Geometry: final body of the model. Coordinates: model frame, mm. A direction names the side the tool comes from. Coordinates: 2 decimals unless noted, no trailing zeros. Order: outer loops, then holes, each group sorted by start corner. A loop starts at its lowest first (then second) coordinate and runs counter-clockwise, first axis right, second up. Notation, with made-up numbers: (-21.5, 59.5) -> (-5.5, 59.5) arc R26 ccw to (-5.5, 87.5) -> close; hole circle Ø9 at (73, 20.25). An arc over 180 degrees is marked (long way). Answer in a Markdown table with one row per item. Add a question column.
1) Ray query, line 1 (X direction, y = 1.8, z = -44); line 2 (Z direction, x = -37, y = 0.65). Return the intervals inside material, ascending. Write a range as from..to.
2) Section query A-A on y = 1.45. Return the cut outline in (x, z) (3 decimals), then the cut area to 3 significant figures.
3) Section query B-B on x = -50.5. Return the cut outline in (y, z) (3 decimals), then the cut area to 3 significant figures.
4) Section query C-C on z = -39.5. Return the cut outline in (x, y) (3 decimals).
5) Contact query for flat-ended pins moving along their axis: P1, Ø1, axis at y = 2, z = -95, coming from the +X side; P2, Ø1, axis at y = 2, z = -81, coming from the -X side; P3, Ø12, axis at x = 17.5, z = -91.5, coming from the -Y side. Output: stop coordinate, or through.
6) Set-up query: faces 1 (the face through (32, 2, 0)), 2 (the face through (59.31, 1.57, 3.24)), 3 (the face through (-6.35, 2, -77)). Return all of +Z, -Z, +X, -X, +Y, -Y with unobstructed straight access to the full face (end or side cutting, diameter ignored); none if empty.
```python
from build123d import *

# Parameters (mm, degrees)
BOSS_EXTRUDE1_DEPTH = 3.175


with BuildPart() as part:
    # Sketch1 → Boss-Extrude1 (new body)
    with BuildSketch(Plane(origin=(0, 0, 0), x_dir=(1, 0, 0), z_dir=(0, 1, 0))):
        with BuildLine():
            Line((-6.35, 0), (-56.134, 0))
            ThreePointArc((-56.134, 0), (-59.309, -3.175), (-56.134, -6.35))
            Line((-56.134, -6.35), (56.134, -6.35))
            ThreePointArc((56.134, -6.35), (59.309, -3.175), (56.134, 0))
            Line((56.134, 0), (6.35, 0))
            Line((6.35, 0), (6.35, 152.4))
            Line((6.35, 152.4), (-6.35, 152.4))
            Line((-6.35, 152.4), (-6.35, 0))
        make_face()
    extrude(amount=BOSS_EXTRUDE1_DEPTH)


solid = part.part
```
Result:
| question | item | result |
|---|---|---|
| 1 | line 1 | -6.35..6.35 |
| 1 | line 2 | 0..6.35 |
| 2 | outline | (-56.134, 0) -> (-6.35, 0) -> (-6.35, -152.4) -> (6.35, -152.4) -> (6.35, 0) -> (56.134, 0) arc R3.175 ccw to (56.134, 6.35) -> (-56.134, 6.35) arc R3.175 ccw to start |
| 2 | area | 2,680 mm2 |
| 3 | outline | (0, 0) -> (3.175, 0) -> (3.175, 6.35) -> (0, 6.35) -> close |
| 3 | area | 20.2 mm2 |
| 4 | outline | (-6.35, 0) -> (6.35, 0) -> (6.35, 3.175) -> (-6.35, 3.175) -> close |
| 5 | P1 | x = 6.35 |
| 5 | P2 | x = -6.35 |
| 5 | P3 | through |
| 6 | face 1 | -Z, +X, +Y, -Y |
| 6 | face 2 | +X, +Y, -Y |
| 6 | face 3 | -Z, -X, +Y, -Y |
